from build123d import *

# Parameters (mm, degrees)
SKETCH1_R          = 3
STEM_HOUSING_DEPTH = 5.6
SKETCH2_R          = 5
BUTTON_HEAD_DEPTH  = 6
FILLET1_R          = 0.5


with BuildPart() as part:
    # Sketch1 → stem housing (new body)
    with BuildSketch(Plane(origin=(0, 0, 0), x_dir=(1, 0, 0), z_dir=(0, 1, 0))):
        with Locations(Location((0, 0, 0), (0, 0, 270))):
            Circle(SKETCH1_R)
        with BuildLine():
            Line((-0.585, 0.885), (-0.585, 2.05))
            Line((-0.585, 2.05), (0.585, 2.05))
            Line((0.585, 2.05), (0.585, 0.885))
            ThreePointArc((0.585, 0.885), (0.672867966, 0.672867966), (0.885, 0.585))
            Line((0.885, 0.585), (2.05, 0.585))
            Line((2.05, 0.585), (2.05, -0.585))
            Line((2.05, -0.585), (0.885, -0.585))
            ThreePointArc((0.885, -0.585), (0.672867966, -0.672867966), (0.585, -0.885))
            Line((0.585, -0.885), (0.585, -2.05))
            Line((0.585, -2.05), (-0.585, -2.05))
            Line((-0.585, -2.05), (-0.585, -0.885))
            ThreePointArc((-0.585, -0.885), (-0.672867966, -0.672867966), (-0.885, -0.585))
            Line((-0.885, -0.585), (-2.05, -0.585))
            Line((-2.05, -0.585), (-2.05, 0.585))
            Line((-2.05, 0.585), (-0.885, 0.585))
            ThreePointArc((-0.885, 0.585), (-0.672867966, 0.672867966), (-0.585, 0.885))
        make_face(mode=Mode.SUBTRACT)
    extrude(amount=STEM_HOUSING_DEPTH)

    # Sketch2 → button head (add)
    with BuildSketch(Plane(origin=(0, 5.6, 0), x_dir=(1, 0, 0), z_dir=(0, 1, 0))):
        with Locations(Location((0, 0, 0), (0, 0, 270))):
            Circle(SKETCH2_R)
    extrude(amount=BUTTON_HEAD_DEPTH)

    # Fillet1
    fillet1_edges = [part.edges().sort_by_distance(p)[0] for p in [
        (0, 11.6, -5),
    ]]
    fillet(fillet1_edges, radius=FILLET1_R)


solid = part.part
Part model, mm, in its own coordinate system. A direction names the side the tool comes from. Coordinates: 2 decimals unless noted, no trailing zeros. Order: outer loops, then holes, each group sorted by start corner. A loop starts at its lowest first (then second) coordinate and runs counter-clockwise, first axis right, second up.
(1) Slice it at C-C, the plane x = 0. Write the cut outline in (y, z), and give its area (3 significant figures).
Check sheet entries:
outline: (0, -3) - (5.6, -3) - (5.6, -5) - (11.1, -5) arc R0.5 ccw to (11.6, -4.5) - (11.6, 4.5) arc R0.5 ccw to (11.1, 5) - (5.6, 5) - (5.6, 3) - (0, 3) - (0, 2.05) - (5.6, 2.05) - (5.6, -2.05) - (0, -2.05) - close
area: 70.5 mm2
(2) Slice it at B-B, the plane z = 0. Write the cut outline in (x, y).
Check sheet entries:
outline: (-5, 5.6) - (-3, 5.6) - (-3, 0) - (-2.05, 0) - (-2.05, 5.6) - (2.05, 5.6) - (2.05, 0) - (3, 0) - (3, 5.6) - (5, 5.6) - (5, 11.1) arc R0.5 ccw to (4.5, 11.6) - (-4.5, 11.6) arc R0.5 ccw to (-5, 11.1) - close
(3) Slice it at A-A, the plane y = 3.25. Write the cut outline in (x, z) (3 decimals).
Check sheet entries:
outline: circle Ø6 at (0, 0); hole (-2.05, -0.585) - (-0.885, -0.585) arc R0.3 cw to (-0.585, -0.885) - (-0.585, -2.05) - (0.585, -2.05) - (0.585, -0.885) arc R0.3 cw to (0.885, -0.585) - (2.05, -0.585) - (2.05, 0.585) - (0.885, 0.585) arc R0.3 cw to (0.585, 0.885) - (0.585, 2.05) - (-0.585, 2.05) - (-0.585, 0.885) arc R0.3 cw to (-0.885, 0.585) - (-2.05, 0.585) - close
(4) Probe L1, parallel to X at y = 3.25, z = 0; L2, parallel to Y at x = 2, z = 0.25; L3, parallel to Z at x = 0.5, y = 5.5. List the from-to ranges inside material, lowest first.
Check sheet entries:
L1: x = -3 to -2.05, 2.05 to 3
L2: y = 5.6 to 11.6
L3: z = -2.96 to -2.05, 2.05 to 2.96
(5) Pin check, flat tips, straight feed: pin 1 Ø4 at (x, z) = (0.5, -0.5) entering from -Y; pin 2 Ø0.9 at (x, y) = (0, 1.5) entering from +Z; pin 3 Ø1 at (x, z) = (2, 3) entering from -Y; pin 4 Ø0.6 at (y, z) = (1.5, 0) entering from -X. Stop position of each tip, or through.
Check sheet entries:
pin 1: stops at y = 0
pin 2: stops at z = 3
pin 3: stops at y = 5.6
pin 4: stops at x = -3
(6) Slice it at D-D, the plane y = 6. Write the cut outline in (x, z).
Check sheet entries:
outline: circle Ø10 at (0, 0)
(7) Tool access for faces 1 (the face through (1.5, 2.8, 0.585)), 2 (the face through (1, 0, -1)): list every direction of +Z, -Z, +X, -X, +Y, -Y with a clear straight run to the whole face (end or side of a thin tool).
Check sheet entries:
face 1: -Y
face 2: +Z, -Z, +X, -X, -Y
